Verification items for the finished model (mm, model axes). Coordinates: 2 decimals unless noted, no trailing zeros. Write each loop counter-clockwise with the first axis right and the second up, starting at its lowest first coordinate (ties: lowest second). Pieces come first, ordered by that corner, then holes. Notation, with made-up numbers: M 56.5,55.5 L 69.5,55.5 A18 cw 69.5,84.5 Z; hole C 87,18.5 d11. An arc over 180 degrees is marked long. One line per item, written item: value.
Autodesk Inventor part; units mm, degrees
ref_plane "YZ Plane" through (0, 0, 0) normal (1, 0, 0) x (0, 1, 0)
ref_plane "XZ Plane" through (0, 0, 0) normal (0, 1, 0) x (-1, 0, 0)
ref_plane "XY Plane" through (0, 0, 0) normal (0, 0, 1) x (1, 0, 0)
sketch "Sketch1" plane through (0, 0, 0) normal (0, 1, 0) x (-1, 0, 0)
  line L0 (0, 0) -> (-25.4, 0)
  line L1 (-25.4, 0) -> (-25.4, 25.4)
  line L2 (-25.4, 25.4) -> (0, 25.4)
  line L3 (0, 25.4) -> (0, 0)
  line L4 (-1.5875, 23.8125) -> (-23.8125, 23.8125)
  line L5 (-23.8125, 23.8125) -> (-23.8125, 1.5875)
  line L6 (-23.8125, 1.5875) -> (-1.5875, 1.5875)
  line L7 (-1.5875, 1.5875) -> (-1.5875, 23.8125)
  dimension "d0" = 25.4
  dimension "d2" = 25.4
  dimension "d3" = 1.5875
extrude "Extrusion1" add sketch "Sketch1" along normal blind 596.9
sketch "Sketch7" plane through (25.4, 0, 0) normal (0, 0, -1) x (-1, 0, 0)
  circle A0 centre (12.7, 552.45) radius 3.3782
  circle A1 centre (12.7, 574.675) radius 3.3782
extrude "Extrusion6" cut sketch "Sketch7" against normal blind 25.4
sketch "Sketch8" plane through (25.4, 0, 25.4) normal (1, 0, 0) x (0, 0, -1)
  circle A0 centre (12.7, 565.15) radius 3.3782
  circle A1 centre (12.7, 542.925) radius 3.3782
  circle A2 centre (12.7, 19.05) radius 3.302
  circle A3 centre (12.7, 38.1) radius 3.302
  arc A4 (25.4, 47.625) -> (22.225, 50.8) centre (22.225, 47.625) ccw
  line L0 (22.225, 50.8) -> (3.175, 50.8)
  arc A5 (3.175, 50.8) -> (0, 47.625) centre (3.175, 47.625) ccw
  line L1 (0, 47.625) -> (0, 4.445)
  line L2 (0, 4.445) -> (25.4, 4.445)
  line L3 (25.4, 47.625) -> (25.4, 4.445)
  arc A6 (22.225, 155.2575) -> (25.4, 158.4325) centre (22.225, 158.4325) ccw
  line L4 (3.175, 155.2575) -> (22.225, 155.2575)
  arc A7 (0, 158.4325) -> (3.175, 155.2575) centre (3.175, 158.4325) ccw
  line L5 (0, 177.4825) -> (0, 158.4325)
  arc A8 (0, 177.4825) -> (-3.175, 180.6575) centre (-3.175, 177.4825) ccw
  line L6 (-7.0866, 180.6575) -> (-3.175, 180.6575)
  line L7 (-7.0866, 180.6575) -> (-7.0866, 244.1575)
  line L8 (-3.175, 244.1575) -> (-7.0866, 244.1575)
  arc A9 (-3.175, 244.1575) -> (0, 247.3325) centre (-3.175, 247.3325) ccw
  line L9 (0, 291.7825) -> (0, 247.3325)
  arc A10 (3.175, 294.9575) -> (0, 291.7825) centre (3.175, 291.7825) ccw
  line L10 (22.225, 294.9575) -> (3.175, 294.9575)
  arc A11 (25.4, 291.7825) -> (22.225, 294.9575) centre (22.225, 291.7825) ccw
  line L11 (25.4, 158.4325) -> (25.4, 291.7825)
  circle A12 centre (12.7, 166.0525) radius 3.302
  circle A13 centre (12.7, 199.7075) radius 3.302
  circle A14 centre (12.7, 225.1075) radius 3.302
  circle A15 centre (12.7, 253.6825) radius 3.302
  circle A16 centre (12.7, 282.2575) radius 3.302
extrude "Extrusion7" cut sketch "Sketch8" against normal blind 25.4 contours A0 | A1 | A2 | A3 | A12 | A14 | A16
sketch "Sketch9" plane through (25.4, 0, 0) normal (0, 0, -1) x (-1, 0, 0)
  circle A0 centre (12.7, 431.8) radius 3.3782
  line L0 (25.4, 440.055) -> (0, 440.055)
  line L1 (0, 368.3) -> (0, 440.055)
  line L2 (25.4, 368.3) -> (0, 368.3)
  line L3 (25.4, 440.055) -> (25.4, 368.3)
  circle A1 centre (12.7, 431.8) radius 3.3782
  circle A2 centre (12.7, 381) radius 3.3782
extrude "Extrusion8" cut sketch "Sketch9" against normal blind 25.4 contours A0 | A2
properties part number "Rebuild Edge Mount 1" material "Aluminum 6061"
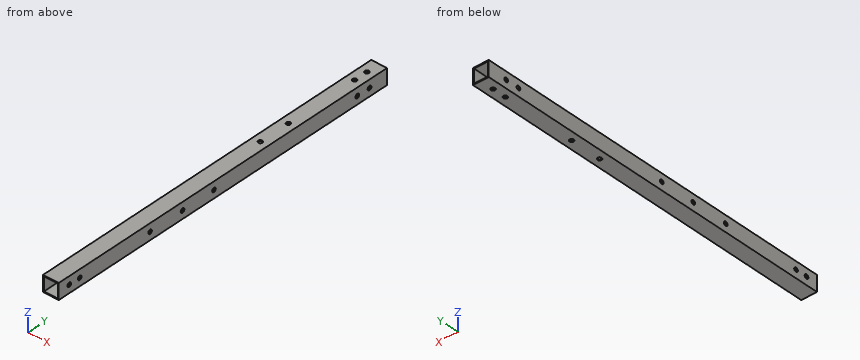
Item 1: Go/stop test with a flat-tipped pin: P1, Ø8, axis at x = 11.5, z = 6.5, coming from the +Y side. Record where the tip stops, or that it passes through.
The answers:
P1: passes through
Item 2: Cross-section at A-A, the plane x = 20. Enter the section's corners in (y, z), and give its area (3 significant figures).
The answers:
outline: M 0,0 L 596.9,0 L 596.9,1.59 L 0,1.59 Z; M 0,23.81 L 596.9,23.81 L 596.9,25.4 L 0,25.4 Z
area: 1,900 mm²
Item 3: Cross-section at B-B, the plane y = 453. Enter the section's corners in (x, z), and give its area (3 significant figures).
The answers:
outline: M 0,0 L 25.4,0 L 25.4,25.4 L 0,25.4 Z; hole M 1.59,1.59 L 23.81,1.59 L 23.81,23.81 L 1.59,23.81 Z
area: 151 mm²
Item 4: Scan lines: line 1 (Y direction, x = 12.7, z = 25); line 2 (X direction, y = 339, z = 10.25). Record each from-to range of solid material in increasing order.
The answers:
line 1: y = 0 to 377.62, 384.38 to 428.42, 435.18 to 549.07, 555.83 to 571.3, 578.05 to 596.9
line 2: x = 0 to 1.59, 23.81 to 25.4
